Autodesk Inventor part; units mm, degrees
ref_plane "YZ Plane" through (0, 0, 0) normal (1, 0, 0) x (0, 1, 0)
ref_plane "XZ Plane" through (0, 0, 0) normal (0, 1, 0) x (-1, 0, 0)
ref_plane "XY Plane" through (0, 0, 0) normal (0, 0, 1) x (1, 0, 0)
sketch "Sketch1" plane through (0, 0, 0) normal (0, 1, 0) x (-1, 0, 0)
  line L0 (-26.035, 33.02) -> (26.035, 33.02)
  line L1 (28.575, 30.48) -> (28.575, -30.48)
  line L2 (26.035, -33.02) -> (-26.035, -33.02)
  line L3 (-28.575, -30.48) -> (-28.575, 30.48)
  line L4 (-28.575, 33.02) -> (28.575, -33.02) construction
  line L5 (28.575, 33.02) -> (-28.575, -33.02) construction
  arc A0 (26.035, -33.02) -> (28.575, -30.48) centre (26.035, -30.48) ccw
  arc A1 (28.575, 30.48) -> (26.035, 33.02) centre (26.035, 30.48) ccw
  arc A2 (-26.035, 33.02) -> (-28.575, 30.48) centre (-26.035, 30.48) ccw
  arc A3 (-28.575, -30.48) -> (-26.035, -33.02) centre (-26.035, -30.48) ccw
  point P0 (0, 0)
  dimension "d0" = 57.15
  dimension "d1" = 66.04
  dimension "d2" = 2.54
extrude "Extrusion1" add sketch "Sketch1" along normal blind 1.6
sketch "Sketch2" plane through (0, 1.6, 0) normal (0, 1, 0) x (1, 0, 0)
  line L0 (25.4, -29.845) -> (-25.4, -29.845) construction
  line L1 (-25.4, -29.845) -> (-25.4, 29.845) construction
  line L2 (-25.4, 29.845) -> (25.4, 29.845) construction
  line L3 (25.4, 29.845) -> (25.4, -29.845) construction
  line L4 (25.4, -29.845) -> (-25.4, 29.845) construction
  line L5 (-25.4, -29.845) -> (25.4, 29.845) construction
  circle A0 centre (-25.4, 29.845) radius 1.4605
  circle A1 centre (-25.4, -29.845) radius 1.4605
  circle A2 centre (25.4, -29.845) radius 1.4605
  circle A3 centre (25.4, 29.845) radius 1.4605
  point P0 (0, 0)
  dimension "d5" = 50.8
  dimension "d6" = 59.69
  dimension "d7" = 2.921
extrude "Extrusion2" cut sketch "Sketch2" against normal through all
sketch "Sketch3" plane through (0, 1.6, 0) normal (0, 1, 0) x (1, 0, 0)
  line L0 (-22.225, 8.89) -> (22.225, 8.89)
  line L1 (22.225, 8.89) -> (22.225, -8.89)
  line L2 (22.225, -8.89) -> (-22.225, -8.89)
  line L3 (-22.225, -8.89) -> (-22.225, 8.89)
  line L4 (-22.225, 8.89) -> (22.225, -8.89) construction
  line L5 (22.225, 8.89) -> (-22.225, -8.89) construction
  line L6 (10.9394, 13.1131) -> (-9.3806, 13.1131)
  line L7 (-9.3806, 13.1131) -> (-9.3806, 29.1151)
  line L8 (-9.3806, 29.1151) -> (10.9394, 29.1151)
  line L9 (10.9394, 29.1151) -> (10.9394, 13.1131)
  line L10 (10.9394, 13.1131) -> (-9.3806, 29.1151) construction
  line L11 (-9.3806, 13.1131) -> (10.9394, 29.1151) construction
  circle A0 centre (-13.6746, -24.0899) radius 4.064
  point P0 (0, 0)
  point P1 (0.7794, 21.1141)
  dimension "d10" = 8.128
  dimension "d11" = 17.78
  dimension "d12" = 44.45
  dimension "d13" = 16.002
  dimension "d14" = 20.32
extrude "Extrusion3" add sketch "Sketch3" along normal blind 19.05
properties part number "pcb"
Source: CAD feature listing. Evaluate the final solid. Frame: model axes, mm. A direction names the side the tool comes from. Coordinates: 2 decimals unless noted, no trailing zeros. Order: outer loops, then holes, each group sorted by start corner. A loop starts at its lowest first (then second) coordinate and runs counter-clockwise, first axis right, second up. Notation, with made-up numbers: M 55.25,-7.75 L 86.25,-7.75 A14 cw 86.25,17.25 Z; hole C -13,4.25 d7. An arc over 180 degrees is marked long. Write each question's results on one line, items separated by ' | '. Start each with the question number.
1. Section C-C, the plane z = -14. Return the cut outline in (x, y) (3 decimals), then the cut area to 3 significant figures.
2. Reachability of faces 5 (the face through (1, 11, -29.115)), 6 (the face through (10.939, 11, -21)), 7 (the face through (22.225, 11, 0)) from +Z, -Z, +X, -X, +Y, -Y: full face, straight path, thin tool, end or side. Return the list, or none.
3. Draft query along X for faces 1 (the face through (1, 11, -13.113)), 2 (the face through (-27.811, 0.789, 32.296)), 3 (the face through (23.94, 0.81, -29.91)), 4 (the face through (28.575, 1, 0)). Return one class per face: +X half, -X half, draft (parallel to the pull), parting line (faces both ways), or undercut.
4. Pin query (flat end, axial travel): pin 1 (4 mm diameter, centred on x = -25.4, z = -29.845, fed in from -Y); pin 2 (4 mm diameter, centred on x = 25.4, z = 29.845, fed in from +Y); pin 3 (5.5 mm diameter, centred on x = -4, y = 12, fed in from +Z); pin 4 (5 mm diameter, centred on y = 10.5, z = -20.5, fed in from +X). Return the tip coordinate at first contact, or that it passes through.
5. Section A-A, the plane x = 1. Return the cut outline in (y, z).
6. Material intervals for L1, parallel to Z at x = -25.4, y = 0.9; L2, parallel to Y at x = 15.5, z = -27.5; L3, parallel to X at y = 13, z = -15, sorted ascending.
7. Section D-D, the plane z = 5.5. Return the cut outline in (x, y) (3 decimals).
8. Section B-B, the plane y = 19.25. Return the cut outline in (x, z) (3 decimals), then the cut area to 3 significant figures.
Solution:
1) outline: M -28.575,0 L 28.575,0 L 28.575,1.6 L 10.939,1.6 L 10.939,20.65 L -9.381,20.65 L -9.381,1.6 L -28.575,1.6 Z | area: 479 mm²
2) face 5: -Z, +X, -X, +Y | face 6: -Z, +X, +Y | face 7: +Z, -Z, +X, +Y
3) face 1: draft | face 2: -X half | face 3: undercut | face 4: +X half
4) pin 1: y = 0 | pin 2: y = 1.6 | pin 3: z = 8.89 | pin 4: x = 10.94
5) outline: M 0,-33.02 L 1.6,-33.02 L 1.6,-29.12 L 20.65,-29.12 L 20.65,-13.11 L 1.6,-13.11 L 1.6,-8.89 L 20.65,-8.89 L 20.65,8.89 L 1.6,8.89 L 1.6,33.02 L 0,33.02 Z
6) L1: -33.02 to -31.31, -28.38 to 28.38, 31.31 to 33.02 | L2: 0 to 1.6 | L3: -9.38 to 10.94
7) outline: M -28.575,0 L 28.575,0 L 28.575,1.6 L 22.225,1.6 L 22.225,20.65 L -22.225,20.65 L -22.225,1.6 L -28.575,1.6 Z
8) outline: M -22.225,-8.89 L 22.225,-8.89 L 22.225,8.89 L -22.225,8.89 Z; C -13.675,24.09 d8.128; M -9.381,-29.115 L 10.939,-29.115 L 10.939,-13.113 L -9.381,-13.113 Z | area: 1,170 mm²
